Could you check a few things on this drawing? It's one solid part, dimensions in mm from its lowest x, y, z. A direction names the side the tool comes from. Give positions to 0.01 mm unless a question says otherwise; leave off trailing zeros. Write each loop counter-clockwise with the first axis right and the second up, starting at its lowest first coordinate (ties: lowest second). Pieces come first, ordered by that corner, then holes.
1. Suppose I cut it at C-C (y = 10.75). Please give me the cut outline in (x, z), and give its area (3 significant figures).
2. Suppose I cut it at D-D (z = 2.05). Please give me the cut outline in (x, y).
3. I'm going to push flat-ended pins straight in: pin 1 (4 mm diameter, centred on x = 7.5, y = 2, fed in from -Z); pin 2 (0.8 mm diameter, centred on x = 6.5, y = 11.5, fed in from +Z); pin 3 (0.6 mm diameter, centred on x = 6.5, y = 10.5, fed in from -Z). Where does each tip first touch, or does it pass through?
4. Suppose I cut it at B-B (z = 3). Please give me the cut outline in (x, y), and give its area (3 significant figures).
5. Suppose I cut it at A-A (x = 5). Please give me the cut outline in (y, z), and give its area (3 significant figures).
6. If I drill on probe 1 along Y at (x, z) = (9.5, 4.3); probe 2 along X at (y, z) = (2.75, 2.85); probe 3 along Y at (x, z) = (4.75, 2.9), over which ranges is the centre line in solid material (lowest first)?
7. On a 3-axis mill with a long thin cutter (end or side, diameter ignored), from which of +Z, -Z, +X, -X, +Y, -Y can I reach the whole of each face in a straight line? I mean the marked faces 1, 2, 3, 4 and 5. Say none if no direction works.
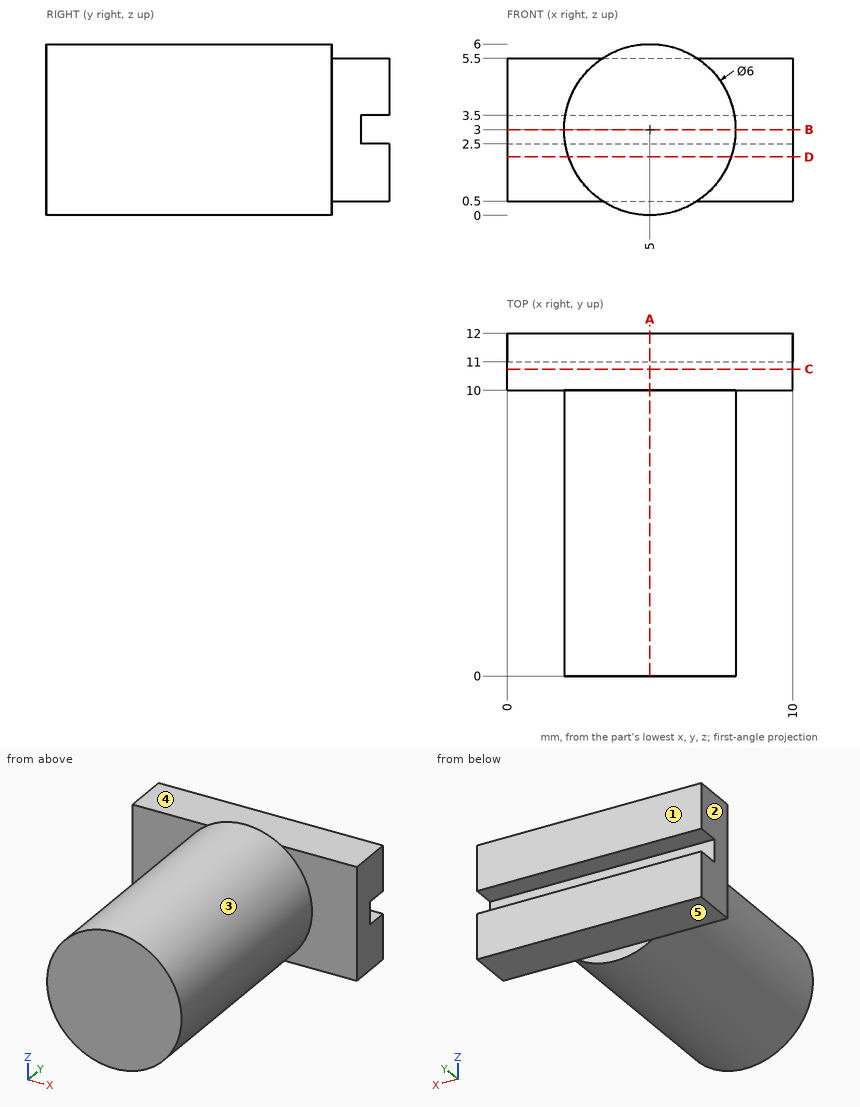
Checks:
1. outline: (0, 0.5) - (10, 0.5) - (10, 5.5) - (0, 5.5) - close
1. area: 50.0 mm2
2. outline: (0, 10) - (2.15, 10) - (2.15, 0) - (7.85, 0) - (7.85, 10) - (10, 10) - (10, 12) - (0, 12) - close
3. pin 1: stops at z = 0.04
3. pin 2: stops at z = 5.5
3. pin 3: stops at z = 0.5
4. outline: (0, 10) - (2, 10) - (2, 0) - (8, 0) - (8, 10) - (10, 10) - (10, 11) - (0, 11) - close
4. area: 70.0 mm2
5. outline: (0, 0) - (10, 0) - (10, 0.5) - (12, 0.5) - (12, 2.5) - (11, 2.5) - (11, 3.5) - (12, 3.5) - (12, 5.5) - (10, 5.5) - (10, 6) - (0, 6) - close
5. area: 69.0 mm2
6. probe 1: y = 10 to 12
6. probe 2: x = 2 to 8
6. probe 3: y = 0 to 11
7. face 1: +Z, -Z, +X, -X, +Y
7. face 2: +Z, -Z, -X, +Y, -Y
7. face 3: -Y
7. face 4: +Z, +X, -X, +Y
7. face 5: -Z, +X, -X, +Y
